Autodesk Inventor part; units mm, degrees
ref_plane "YZ Plane" through (0, 0, 0) normal (1, 0, 0) x (0, 1, 0)
ref_plane "XZ Plane" through (0, 0, 0) normal (0, 1, 0) x (-1, 0, 0)
ref_plane "XY Plane" through (0, 0, 0) normal (0, 0, 1) x (1, 0, 0)
sketch "Sketch2" plane through (0, 0, 0) normal (0, 0, 1) x (1, 0, 0)
  line L0 (0, 0) -> (-9.9, 0)
  line L1 (-4.95, 0) -> (-4.95, 2.5)
  line L2 (-4.95, 0) -> (-2.45, 0) construction
  circle A0 centre (-4.95, 5) radius 2.5
  line L3 (-4.95, 7.5) -> (32.05, 7.5) construction
  line L4 (0, 44.5) -> (0, 0)
  line L5 (0, 0) -> (-9.9, 0)
  line L6 (-9.9, 0) -> (-9.9, 44.5)
  line L7 (0, 45.5) -> (0, 0)
  line L8 (0, 0) -> (-9.9, 0)
  line L9 (-9.9, 0) -> (-9.9, 45.5)
  line L10 (-4.95, 7.5) -> (66.05, 7.5) construction
  line L11 (0, 0) -> (-9.9, 0)
  line L12 (-9.9, 0) -> (-9.9, 88)
  line L13 (-9.9, 88) -> (0, 88)
  line L14 (0, 88) -> (0, 0)
  dimension "d35" = 5
  dimension "d33" = 2.5
  dimension "d34" = 90
  dimension "d46" = 88
extrude "Extrusion6" add sketch "Sketch2" along normal blind 5
properties part number "Elbow_Cube_Holder_TestFit_V2"
CAD build for the part. Positions are in the model's coordinates, mm. Give positions to 0.01 mm unless a question says otherwise; leave off trailing zeros. Write each loop counter-clockwise with the first axis right and the second up, starting at its lowest first coordinate (ties: lowest second). Pieces come first, ordered by that corner, then holes. Notation, with made-up numbers: M -1,49 L 31,49 A27 ccw 31,73 Z; hole C 77.5,13.25 d2. An arc over 180 degrees is marked long. Put each result on its own line as item: value. Start each with the question number.
(1) Flat gauge pin, fed straight in: pin 1 Ø1.5 at (y, z) = (26.5, 3) entering from +X. Where does the tip first touch, or does it go through?
(2) Probe L1, parallel to Y at x = -4.95, z = 1.7; L2, parallel to X at y = 5, z = 3; L3, parallel to Y at x = -5.75, z = 4.7. List the from-to ranges inside material, lowest first.
(3) Band-saw the part on A-A, the plane y = 5. Write the cut outline in (x, z), and give its area (3 significant figures).
(4) Band-saw the part on B-B, the plane x = -4.95. Write the cut outline in (y, z), and give its area (3 significant figures).
(5) Mould opens along X. For faces 1 (the face through (-5, 45, 0)), 2 (the face through (-9.9, 43, 2)), 3 (the face through (-2.565, 4.249, 2.465)) say: +X half, -X half, draft (parallel to the pull), parting line (faces both ways), or undercut.
(6) Band-saw the part on C-C, the plane z = 2.1. Write the cut outline in (x, y).
Response values:
1. pin 1: stops at x = 0
2. L1: y = 0 to 2.5, 7.5 to 88
2. L2: x = -9.9 to -7.45, -2.45 to 0
2. L3: y = 0 to 2.63, 7.37 to 88
3. outline: M -9.9,0 L -7.45,0 L -7.45,5 L -9.9,5 Z; M -2.45,0 L 0,0 L 0,5 L -2.45,5 Z
3. area: 24.5 mm2
4. outline: M 0,0 L 2.5,0 L 2.5,5 L 0,5 Z; M 7.5,0 L 88,0 L 88,5 L 7.5,5 Z
4. area: 415 mm2
5. face 1: draft
5. face 2: -X half
5. face 3: undercut
6. outline: M -9.9,0 L 0,0 L 0,88 L -9.9,88 Z; hole C -4.95,5 d5
